Geometry: final body of the model. Coordinates: model frame, mm. Coordinates: 2 decimals unless noted, no trailing zeros. Write each loop counter-clockwise with the first axis right and the second up, starting at its lowest first coordinate (ties: lowest second). Pieces come first, ordered by that corner, then holes.
from build123d import *

# Parameters (mm, degrees)
RESSALTO_EXTRUS_O3_DEPTH = 40
ESBO_O8_R                = 1.5
CORTE_EXTRUS_O1_DEPTH    = 40
ESBO_O9_R                = 1.5
CORTE_EXTRUS_O2_DEPTH    = 26


with BuildPart() as part:
    # Esboço7 → Ressalto-extrusão3 (new body)
    with BuildSketch(Plane.XY):
        with BuildLine():
            Line((103.35727616, -256.335501283), (87.35727616, -256.335501283))
            ThreePointArc((87.35727616, -256.335501283), (84.528849035, -255.163928408), (83.35727616, -252.335501283))
            Line((83.35727616, -252.335501283), (83.35727616, -236.335501283))
            Line((83.35727616, -236.335501283), (83.35727616, -231.335501283))
            ThreePointArc((83.35727616, -231.335501283), (101.034945689, -238.657831753), (108.35727616, -256.335501283))
            Line((108.35727616, -256.335501283), (103.35727616, -256.335501283))
        make_face()
    extrude(amount=RESSALTO_EXTRUS_O3_DEPTH)

    # Esboço8 → Corte-extrusão1 (cut)
    with BuildSketch(Plane(origin=(0, 0, 0), x_dir=(-1, 0, 0), z_dir=(0, 0, -1))):
        with Locations((-88.35727616, -238.335501283)):
            Circle(ESBO_O8_R)
        with Locations((-101.35727616, -251.335501283)):
            Circle(ESBO_O8_R)
    extrude(amount=-CORTE_EXTRUS_O1_DEPTH, mode=Mode.SUBTRACT)

    # Esboço9 → Corte-extrusão2 (cut, through all)
    with BuildSketch(Plane.XZ.offset(256.335501283)):
        with Locations((95.85727616, 8)):
            Circle(ESBO_O9_R)
        with Locations((95.85727616, 18)):
            Circle(ESBO_O9_R)
        with Locations((95.85727616, 22)):
            Circle(ESBO_O9_R)
        with Locations((95.85727616, 32)):
            Circle(ESBO_O9_R)
    extrude(amount=-CORTE_EXTRUS_O2_DEPTH, mode=Mode.SUBTRACT)


solid = part.part
Item 1: Section C-C, the plane y = -244.25. Output: boundary loops of the cut face in (x, z).
Derived:
outline: (83.36, 0) - (105.24, 0) - (105.24, 40) - (83.36, 40) - close; hole circle Ø3 at (95.86, 8); hole circle Ø3 at (95.86, 18); hole circle Ø3 at (95.86, 22); hole circle Ø3 at (95.86, 32)
Item 2: Material intervals for probe 1 along X at (y, z) = (-250.75, 7); probe 2 along X at (y, z) = (-251.5, 7.5); probe 3 along X at (y, z) = (-237.5, 28), sorted ascending.
Derived:
probe 1: x = 83.36 to 94.74, 96.98 to 99.98, 102.74 to 107.73
probe 2: x = 83.36 to 94.44, 97.27 to 99.87, 102.85 to 107.89
probe 3: x = 83.36 to 87.11, 89.6 to 99.8
Item 3: Pin query (flat end, axial travel): pin 1 (8 mm diameter, centred on y = -248, z = 35, fed in from +X); pin 2 (8 mm diameter, centred on x = 104, z = 15, fed in from +Y); pin 3 (2.5 mm diameter, centred on x = 95.86, z = 18, fed in from +Y); pin 4 (4 mm diameter, centred on x = 95.86, z = 22, fed in from +Y). Return the tip coordinate at first contact, or that it passes through.
Derived:
pin 1: stops at x = 107.98
pin 2: stops at y = -237.68
pin 3: passes through
pin 4: stops at y = -233.65
Item 4: Pull-direction query (X, two-part tool) for faces 1 (the flat face through (98, -256.336, 20)), 2 (the cylindrical face through (84.56, -255.195, 19.72)), 3 (the cylindrical face through (101.68, -252.8, 19.72)); classes: released by +X, released by -X, zero draft, split by the parting line, or undercut.
Derived:
face 1: zero draft
face 2: released by -X
face 3: undercut
Item 5: Section B-B, the plane z = 22. Output: boundary loops of the cut face in (x, y).
Derived:
outline: (83.36, -252.34) arc R4 ccw to (87.36, -256.34) - (94.36, -256.34) - (94.36, -233.89) arc R25 ccw to (83.36, -231.34) - close; (97.36, -256.34) - (108.36, -256.34) arc R25 ccw to (97.36, -235.62) - close; hole circle Ø3 at (88.36, -238.34); hole circle Ø3 at (101.36, -251.34)
Item 6: Section D-D, the plane z = 28. Output: boundary loops of the cut face in (x, y), plus the area to 3 significant figures.
Derived:
outline: (83.36, -252.34) arc R4 ccw to (87.36, -256.34) - (108.36, -256.34) arc R25 ccw to (83.36, -231.34) - close; hole circle Ø3 at (88.36, -238.34); hole circle Ø3 at (101.36, -251.34)
area: 473 mm2
Item 7: Section A-A, the plane x = 101.5. Output: boundary loops of the cut face in (y, z), plus the area to 3 significant figures.
Derived:
outline: (-256.34, 0) - (-252.83, 0) - (-252.83, 40) - (-256.34, 40) - close; (-249.84, 0) - (-239.14, 0) - (-239.14, 40) - (-249.84, 40) - close
area: 569 mm2
